Could you check a few things on this model? Use its own coordinates, in mm. A direction names the side the tool comes from. Give positions to 0.01 mm unless a question says otherwise; leave off trailing zeros. Write each loop counter-clockwise with the first axis right and the second up, starting at its lowest first coordinate (ties: lowest second). Pieces come first, ordered by that corner, then holes. Notation, with made-up numbers: M 9.25,7 L 49.25,7 A21 ccw 49.25,37 Z; hole C 18.25,68 d3. An arc over 180 degrees is marked long. One line per item, written item: value.
Autodesk Inventor part; units mm, degrees
ref_plane "YZ Plane" through (0, 0, 0) normal (1, 0, 0) x (0, 1, 0)
ref_plane "XZ Plane" through (0, 0, 0) normal (0, 1, 0) x (-1, 0, 0)
ref_plane "XY Plane" through (0, 0, 0) normal (0, 0, 1) x (1, 0, 0)
sketch "スケッチ1" plane through (0, 0, 0) normal (0, 0, 1) x (1, 0, 0)
  line L0 (-30, 15) -> (30, 15)
  line L1 (30, 15) -> (30, -15)
  line L2 (30, -15) -> (-30, -15)
  line L3 (-30, -15) -> (-30, 15)
  line L4 (-28, 13) -> (28, 13)
  line L5 (28, 13) -> (28, -13)
  line L6 (28, -13) -> (-28, -13)
  line L7 (-28, -13) -> (-28, 13)
  point P0 (0, 0)
  dimension "d0" = 60
  dimension "d2" = 2
  dimension "d3" = 2
  dimension "d4" = 30
  dimension "d5" = 15
  dimension "d6" = 30
  dimension "d7" = 56
  dimension "d8" = 26
extrude "押し出し1" add sketch "スケッチ1" against normal blind 60
sketch "スケッチ2" plane through (-30, 15, 0) normal (0, 1, 0) x (1, 0, 0)
  line L0 (0, 0) -> (60, 0)
  line L1 (60, 0) -> (60, 60)
  line L2 (0, 60) -> (60, 60)
  line L3 (60, 60) -> (60, 15)
  line L4 (60, 15) -> (0, 15)
  line L5 (0, 15) -> (0, 60)
  point P0 (30, 0)
  dimension "d11" = 15
extrude "押し出し2" cut sketch "スケッチ2" against normal blind 2
sketch "スケッチ3" plane through (30, -15, 0) normal (1, 0, 0) x (0, 0, -1)
  line L0 (0, 0) -> (60, 0)
  line L1 (60, 28) -> (60, 0)
  arc A0 (50, 22) -> (50, 14) centre (50, 18) ccw
  line L2 (50, 22) -> (60, 22)
  line L3 (50, 14) -> (60, 14)
  point P0 (0, 15)
  dimension "d14" = 8
  dimension "d16" = 10
  dimension "d17" = 18
extrude "押し出し3" cut sketch "スケッチ3" against normal blind 60
sketch "スケッチ4" plane through (30, -15, 0) normal (1, 0, 0) x (0, 0, -1)
  line L0 (50, 22) -> (60, 22)
  line L1 (60, 28) -> (60, 22)
  line L2 (60, 14) -> (60, 0)
  line L3 (60, 14) -> (50, 14)
  arc A0 (50, 22) -> (50, 14) centre (50, 18) ccw
  arc A1 (50, 23) -> (50, 13) centre (50, 18) ccw
  line L4 (50, 23) -> (60, 23)
  line L5 (50, 13) -> (60, 13)
  point P0 (0, 15)
  dimension "d20" = 10
extrude "押し出し4" cut sketch "スケッチ4" against normal blind 2
sketch "スケッチ5" plane through (30, -15, 0) normal (1, 0, 0) x (0, 0, -1)
  line L0 (60, 28) -> (60, 23)
  arc A0 (50, 23) -> (50, 13) centre (50, 18) ccw
  circle A1 centre (50, 25) radius 1
  point P0 (0, 15)
  dimension "d24" = 2
  dimension "d26" = 7
  dimension "d27" = 10
hole "穴1" at (30, 10, -50) direction (-1, 0, 0) diameter 2 end through all
pattern_circular "円形状パターン1" count 5 over 180 about axis through (30, 3, -50) along (1, 0, 0) of "穴1"
sketch "スケッチ6" plane through (-30, -15, 0) normal (0, -1, 0) x (1, 0, 0)
  line L0 (60, 0) -> (0, 0)
  line L1 (0, 0) -> (0, -60)
  circle A0 centre (30, -30) radius 5
  point P0 (30, 0)
  dimension "d38" = 10
  dimension "d40" = 30
  dimension "d41" = 30
hole "穴2" at (0, -15, -30) direction (0, 1, 0) diameter 10 end through all
sketch "スケッチ7" plane through (-30, -15, 0) normal (0, -1, 0) x (1, 0, 0)
  circle A0 centre (30, -30) radius 5
  line L0 (60, 0) -> (60, -60)
  circle A1 centre (30, -23) radius 1
  point P0 (30, 0)
  dimension "d49" = 2
  dimension "d51" = 7
  dimension "d52" = 30
hole "穴3" at (0, -15, -23) direction (0, 1, 0) diameter 2 depth 2 tip angle 118
pattern_circular "円形状パターン2" count 8 over 360 about axis through (0, 75, -30) along (0, -1, 0) of "穴3"
sketch "スケッチ8" plane through (-30, 13, 0) normal (0, 1, 0) x (1, 0, 0)
  line L0 (58, 15) -> (58, 60)
  line L1 (60, 15) -> (58, 15)
  line L2 (60, 60) -> (60, 15)
  line L3 (58, 60) -> (60, 60)
  line L4 (0, 60) -> (2, 60)
  line L5 (2, 60) -> (2, 15)
  line L6 (2, 15) -> (0, 15)
  line L7 (0, 15) -> (0, 60)
  line L8 (0, 15) -> (0, 60)
  point P0 (30, 0)
  dimension "d64" = 2
  dimension "d66" = 56
  dimension "d67" = 45
  dimension "d68" = 0
extrude "押し出し5" add sketch "スケッチ8" along normal blind 2
properties part number "Arm_Bracket"
1) On a 3-axis mill with a long thin cutter (end or side, diameter ignored), from which of +Z, -Z, +X, -X, +Y, -Y can I reach the whole of each face in a straight line? I mean faces 1 (the face through (29, -2, -55)), 2 (the face through (-29.01, 8.41, -45.94)), 3 (the face through (-29, 7, -55)), 4 (the face through (0, 13, -7)), 5 (the face through (0, 15, -12)). Say none if no direction works.
Outcome:
face 1: -Z, +X
face 2: +X, -X
face 3: -Z, +X, -X
face 4: +Z, -Z
face 5: +Z, -Z, +X, -X, +Y
2) If we section it at B-B, the plane z = -43: Write out the boundary of the cut face in (x, y).
Outcome:
outline: M -30,-15 L 30,-15 L 30,2 L 28,2 L 28,-13 L -28,-13 L -28,2 L -30,2 Z; M -30,4 L -28,4 L -28,15 L -30,15 Z; M 28,4 L 30,4 L 30,15 L 28,15 Z
3) If we section it at A-A, the plane x = 7: Write out the boundary of the cut face in (y, z), then the cut area to 3 significant figures.
Outcome:
outline: M -15,-60 L -13,-60 L -13,-31 L -15,-31 Z; M -15,-29 L -13,-29 L -13,0 L -15,0 Z; M 13,-15 L 15,-15 L 15,0 L 13,0 Z
area: 146 mm^2
4) We'd pull the mould along Z, two halves only. Please class faces 6 (the face through (29, 10, -51)), 7 (the face through (-5.166, -13.986, -26.027)), 8 (the face through (29, 3, -45)), 9 (the face through (-5.8, -13, -29.6)): pulls with the +Z half, pulls with the -Z half, needs draft (parallel to the pull), parting line crosses it, or undercut.
Outcome:
face 6: undercut
face 7: undercut
face 8: pulls with the -Z half
face 9: needs draft
5) Please list where these lines run through material, in increasing order: L1, parallel to Y at x = -29.5, z = -50; L2, parallel to Y at x = -7, z = -10.5; L3, parallel to X at y = 8.75, z = -40. Write a range as from..to.
Outcome:
L1: y = -15..-5, -3..-1, 7..9, 11..15
L2: y = -15..-13, 13..15
L3: x = -30..-28, 28..30
6) If we section it at C-C, the plane y = -4: Write out the boundary of the cut face in (x, z), then the cut area to 3 significant figures.
Outcome:
outline: M -30,-60 L -28,-60 L -28,-51 L -30,-51 Z; M -30,-49 L -28,-49 L -28,0 L -30,0 Z; M 28,-60 L 30,-60 L 30,-51 L 28,-51 Z; M 28,-49 L 30,-49 L 30,0 L 28,0 Z
area: 232 mm^2
7) I'm going to push flat-ended pins straight in: pin 1 (2.5 mm diameter, centred on y = 7.95, z = -45.05, fed in from +X); pin 2 (1.2 mm diameter, centred on y = 10, z = -50, fed in from -X); pin 3 (12 mm diameter, centred on x = 9.5, z = -47.5, fed in from +Y). Where does each tip first touch, or does it pass through?
Outcome:
pin 1: stops at x = 30
pin 2: passes through
pin 3: stops at y = -13
8) If we section it at D-D, the plane z = -14: Write out the boundary of the cut face in (x, y), then the cut area to 3 significant figures.
Outcome:
outline: M -30,-15 L 30,-15 L 30,15 L -30,15 Z; hole M -28,-13 L 28,-13 L 28,13 L -28,13 Z
area: 344 mm^2
